Model file for the job. Use its own axes, mm. A direction names the side the tool comes from. Coordinates: 2 decimals unless noted, no trailing zeros. Order: outer loops, then holes, each group sorted by start corner. A loop starts at its lowest first (then second) coordinate and runs counter-clockwise, first axis right, second up. Notation, with made-up numbers: (-10.5, 47) -> (16.5, 47) arc R13 ccw to (16.5, 56) -> close; hole circle Ø1 at (53, -6.75). An arc over 180 degrees is marked (long way). Use CSV: the item, a comma, the result in double quotes. Start each with the question number.
(1) Pin check, flat tips, straight feed: pin 1 Ø3 at (x, z) = (1, 16) entering from -Y; pin 2 Ø1.4 at (x, z) = (-0.5, -25) entering from -Y; pin 3 Ø3 at (x, z) = (-0.5, 24.5) entering from +Y; pin 4 Ø3 at (x, z) = (0, 0) entering from +Y. Stop position of each tip, or through.
(2) Probe L1, parallel to Z at x = 0, y = 2.75; L2, parallel to X at y = 3, z = 25; L3, parallel to Z at x = -1, y = -4.25. List the from-to ranges inside material, lowest first.
(3) Cut at C-C on x = 0. Give the number of separate pieces and of enclosed holes in the cut face, plus the area to 3 significant figures.
(4) Cut at D-D on z = -20. Write the cut outline in (x, y), plus the area to 4 significant figures.
(5) Cut at B-B on y = -2.5. Write the cut outline in (x, z).
(6) Cut at A-A on z = 0. Write the cut outline in (x, y).
(7) Pull direction Y, two halves, no side cores. Call faces 4 (the cylindrical face through (-0.488, -2.224, -22.804)), 5 (the cylindrical face through (-0.52, -4.197, 27.343)), 6 (the flat face through (-3, 3.75, 0)): pulls with the +Y half, pulls with the -Y half, needs draft (parallel to the pull), parting line crosses it, or undercut.
(8) Tool access for faces 1 (the cylindrical face through (2.25, 1.85, 17.83)), 2 (the flat face through (-1, -4.4, -26)), 3 (the cylindrical face through (-2.578, 2.99, -0.338)): list every direction of +Z, -Z, +X, -X, +Y, -Y with a clear straight run to the whole face (end or side of a thin tool).
Autodesk Inventor part; units mm, degrees
ref_plane "YZ Plane" through (0, 0, 0) normal (1, 0, 0) x (0, 1, 0)
ref_plane "XZ Plane" through (0, 0, 0) normal (0, 1, 0) x (-1, 0, 0)
ref_plane "XY Plane" through (0, 0, 0) normal (0, 0, 1) x (1, 0, 0)
sketch "Sketch1" plane through (0, 0, 0) normal (0, 1, 0) x (-1, 0, 0)
  line L0 (0, 25) -> (0, -25) construction
  line L1 (-3.5, 25) -> (-3.5, -25)
  line L2 (3.5, -25) -> (3.5, 25)
  arc A0 (3.5, 25) -> (-3.5, 25) centre (0, 25) ccw
  arc A1 (-3.5, -25) -> (3.5, -25) centre (0, -25) ccw
  point P0 (0, 0)
  point P1 (0, 0)
  dimension "d0" = 50
  dimension "d1" = 7
extrude "Extrusion1" add sketch "Sketch1" along normal blind 3.75
sketch "Sketch2" plane through (0, 3.75, 0) normal (0, 1, 0) x (1, 0, 0)
  arc A0 (3.5, 25) -> (-3.5, 25) centre (0, 25) ccw
  line L0 (-3.5, 25) -> (-3.5, -25)
  arc A1 (-3.5, -25) -> (3.5, -25) centre (0, -25) ccw
  line L1 (3.5, -25) -> (3.5, 25)
  circle A2 centre (0, 25) radius 1.5
  circle A3 centre (0, -25) radius 1.5
  arc A4 (-3.5, -25) -> (3.5, -25) centre (0, -25) ccw
  point P0 (0, 0)
  dimension "d38" = 3
  dimension "d39" = 3
sketch "Sketch3" plane through (0, 0, 0) normal (0, -1, 0) x (1, 0, 0)
  arc A0 (-3.5, -25) -> (3.5, -25) centre (0, -25) ccw
  line L0 (3.5, 25) -> (3.5, -25)
  arc A1 (3.5, 25) -> (-3.5, 25) centre (0, 25) ccw
  line L1 (-3.5, -25) -> (-3.5, 25)
  circle A2 centre (0, 0) radius 2.5
  circle A3 centre (0, 0) radius 1.2
  dimension "d11" = 5
  dimension "d14" = 2.4
extrude "Extrusion2" add sketch "Sketch3" along normal blind 7 contours A2 | A3
sketch "Sketch5" plane through (0, -7, 0) normal (0, -1, 0) x (1, 0, 0)
  point P0 (0, 0)
  point P1 (0, 0)
hole "Hole2" at (0, -7, 0) direction (0, 1, 0) diameter 2.4 depth 10 tip angle 118
sketch "Sketch6" plane through (0, 3.75, 0) normal (0, 1, 0) x (1, 0, 0)
  point P0 (0, 0)
  point P1 (0, 0)
hole "Hole3" at (0, 3.75, 0) direction (0, -1, 0) diameter 5.2 depth 1.5
sketch "Sketch8" plane through (0, 0, 0) normal (0, -1, 0) x (1, 0, 0)
  circle A0 centre (0, 0) radius 2.5
  arc A1 (-3.5, -25) -> (3.5, -25) centre (0, -25) ccw
  line L0 (3.5, 25) -> (3.5, -25)
  arc A2 (3.5, 25) -> (-3.5, 25) centre (0, 25) ccw
  line L1 (-3.5, -25) -> (-3.5, 25)
  line L2 (3.5, 25) -> (3.5, -25)
  line L3 (3.5, -13) -> (3.5, -17) construction
  line L4 (2, -13) -> (2, -17)
  line L5 (5, -17) -> (5, -13)
  arc A3 (5, -13) -> (2, -13) centre (3.5, -13) ccw
  arc A4 (2, -17) -> (5, -17) centre (3.5, -17) ccw
  line L6 (-5.2, 0) -> (6.7, 0)
  line L7 (3.5, 13) -> (3.5, 17) construction
  line L8 (2, 13) -> (2, 17)
  line L9 (5, 17) -> (5, 13)
  arc A5 (2, 13) -> (5, 13) centre (3.5, 13) ccw
  arc A6 (5, 17) -> (2, 17) centre (3.5, 17) ccw
  point P0 (3.5, -15)
  point P1 (3.5, -18.5)
  point P2 (3.5, -11.5)
  point P3 (3.5, 15)
  point P4 (3.5, 11.5)
  point P5 (3.5, 18.5)
  dimension "d32" = 4
  dimension "d33" = 3
  dimension "d34" = 15
extrude "Extrusion4" cut sketch "Sketch8" against normal through all contours A5 L8 A6 L0 | L0 A4 L4 A3
fillet "Fillet1" radius 1 4 edges at (3.5, 1.875, -11.5) (3.5, 1.875, -18.5) (3.5, 1.875, 18.5) (3.5, 1.875, 11.5)
extrude "Extrusion5" [suppressed]
sketch "Sketch9" plane through (0, 9.55, -25) normal (0, 1, 0) x (1, 0, 0)
  circle A0 centre (0, 0) radius 1.5
  circle A1 centre (0, -50) radius 1.5
  circle A2 centre (0, -50) radius 1.5
  circle A3 centre (0, -50) radius 1.85
  circle A4 centre (0, 0) radius 1.5
  circle A5 centre (0, 0) radius 1.85
  point P0 (0, -25)
  dimension "d42" = 3.7
  dimension "d43" = 3.7
extrude "Extrusion6" [suppressed]
chamfer "Chamfer1" [suppressed]
fillet "Fillet2" [suppressed]
sketch "Sketch10" plane through (0, 0, 0) normal (0, -1, 0) x (1, 0, 0)
  arc A0 (3.5, 25) -> (-3.5, 25) centre (0, 25) ccw
  arc A1 (-3.5, -25) -> (3.5, -25) centre (0, -25) ccw
  circle A2 centre (0, 25) radius 2.25
  circle A3 centre (0, -25) radius 2.25
  point P0 (0, 0)
  dimension "d50" = 4.5
extrude "Extrusion7" add sketch "Sketch10" along normal blind 4
sketch "Sketch11" plane through (0, -4, 25) normal (0, -1, 0) x (1, 0, 0)
  circle A0 centre (0, 0) radius 2.25
  circle A1 centre (0, -50) radius 2.25
  circle A2 centre (0, 0) radius 2.4
  circle A3 centre (0, -50) radius 2.4
  point P0 (0, -25)
  dimension "d54" = 4.8
  dimension "d70" = 4.5
extrude "Extrusion8" add sketch "Sketch11" along normal blind 0.4 contours A0 | A1 | A2 | A3
fillet "Fillet3" radius 0.4 2 edges at (-2.25, -4, 25) (-2.25, -4, -25)
fillet "Fillet4" radius 0.8 3 edges at (-2.25, 0, 25) (-2.25, 0, -25) (-2.5, 0, 0)
sketch "Sketch13" plane through (0, 3.75, 0) normal (0, 1, 0) x (1, 0, 0)
  circle A0 centre (0, -25) radius 2.4
  circle A1 centre (0, 25) radius 2.25
  circle A2 centre (0, -25) radius 3.05
  point P0 (0, 0)
hole "Hole4" at (0, 3.75, 25) at (0, 3.75, -25) direction (0, -1, 0) diameter 2.2 end through all counterbore diameter 3.6 counterbore depth 1.5
equation "\"d43\" = d42"
properties part number "ActuatorLink"
Outcome:
1,pin 1,"y = 0"
1,pin 2,"y = -4.4"
1,pin 3,"y = 3.75"
1,pin 4,"y = 2.25"
2,L1,"-28.5 to -26.8, -23.2 to -2.6, 2.6 to 23.2, 26.8 to 28.5"
2,L2,"-3.5 to -1.8, 1.8 to 3.5"
2,L3,"-27.18 to -25.46, -24.54 to -22.82, -2.29 to -0.66, 0.66 to 2.29, 22.82 to 24.54, 25.46 to 27.18"
3,separate pieces,"4"
3,enclosed holes,"0"
3,area,"219 mm2"
4,outline,"(-3.5, 0) -> (3.5, 0) -> (3.5, 3.75) -> (-3.5, 3.75) -> close"
4,area,"26.25 mm2"
5,outline,"circle Ø5 at (0, 0); circle Ø4.5 at (0, -25); circle Ø4.5 at (0, 25); hole circle Ø2.4 at (0, 0); hole circle Ø2.2 at (0, -25); hole circle Ø2.2 at (0, 25)"
6,outline,"(-3.5, 0) -> (-3.3, 0) arc R0.8 cw to (-2.5, -0.8) -> (-2.5, -7) -> (-1.2, -7) -> (-1.2, 2.25) -> (-2.6, 2.25) -> (-2.6, 3.75) -> (-3.5, 3.75) -> close; (1.2, -7) -> (2.5, -7) -> (2.5, -0.8) arc R0.8 cw to (3.3, 0) -> (3.5, 0) -> (3.5, 3.75) -> (2.6, 3.75) -> (2.6, 2.25) -> (1.2, 2.25) -> close"
7,face 4,"undercut"
7,face 5,"needs draft"
7,face 6,"pulls with the +Y half"
8,face 1,"+X, +Y, -Y"
8,face 2,"-Z, +X, -X, -Y"
8,face 3,"+Y"
